from build123d import *

# Parameters (mm, degrees)
SKETCH1_R           = 5.0927
BOSS_EXTRUDE1_DEPTH = 5.2578
SKETCH2_R           = 2.3495
CUT_EXTRUDE1_DEPTH  = 9.917154671
SKETCH3_R           = 4.2037
CUT_EXTRUDE2_DEPTH  = 4.4958
CUT_EXTRUDE3_DEPTH  = 4.4958
BOSS_EXTRUDE2_START = 2.54
BOSS_EXTRUDE2_DEPTH = 2.54


with BuildPart() as part:
    # Sketch1 → Boss-Extrude1 (new body)
    with BuildSketch(Plane(origin=(0, 0, 0), x_dir=(1, 0, 0), z_dir=(0, 1, 0))):
        with Locations(Location((0, 0, 0), (0, 0, 270))):
            Circle(SKETCH1_R)
    extrude(amount=BOSS_EXTRUDE1_DEPTH)

    # Sketch2 → Cut-Extrude1 (cut, through all)
    with BuildSketch(Plane(origin=(0, 5.2578, 0), x_dir=(1, 0, 0), z_dir=(0, 1, 0))):
        with Locations(Location((0, 0, 0), (0, 0, 270))):
            Circle(SKETCH2_R)
    extrude(amount=-CUT_EXTRUDE1_DEPTH, mode=Mode.SUBTRACT)

    # Sketch3 → Cut-Extrude2 (cut)
    with BuildSketch(Plane.XZ):
        with Locations(Location((0, 0, 0), (0, 0, 270))):
            Circle(SKETCH3_R)
    extrude(amount=-CUT_EXTRUDE2_DEPTH, mode=Mode.SUBTRACT)

    # Sketch5 → Cut-Extrude3 (cut)
    with BuildSketch(Plane.XZ):
        with BuildLine():
            Line((0, 0), (4.51728007, 2.351547163))
            ThreePointArc((4.51728007, 2.351547163), (0, 5.0927), (-4.51728007, 2.351547163))
            Line((-4.51728007, 2.351547163), (0, 0))
        make_face()
    extrude(amount=-CUT_EXTRUDE3_DEPTH, mode=Mode.SUBTRACT)

    # Sketch4 → Boss-Extrude2 (add)
    with BuildSketch(Plane(origin=(0, 5.2578, 0), x_dir=(1, 0, 0), z_dir=(0, 1, 0)).offset(BOSS_EXTRUDE2_START)):
        with BuildLine():
            Line((4.332897797, 4.7285282), (1.587299193, 1.732233103))
            ThreePointArc((1.587299193, 1.732233103), (-0.306671289, 2.329399702), (-1.981548202, 1.26238543))
            Line((-1.981548202, 1.26238543), (-5.409091038, 3.445971038))
            ThreePointArc((-5.409091038, 3.445971038), (-0.837129734, 6.358631618), (4.332897797, 4.7285282))
        make_face()
    extrude(amount=-BOSS_EXTRUDE2_DEPTH)


solid = part.part
Input: part model. Units: mm. Frame: model coordinates. A direction names the side the tool comes from. Give positions to 0.01 mm unless a question says otherwise; leave off trailing zeros. Write each loop counter-clockwise with the first axis right and the second up, starting at its lowest first coordinate (ties: lowest second). Pieces come first, ordered by that corner, then holes.
Q1. Pull-direction query (X, two-part tool) for faces 6 (the face through (-0.91, 6.55, -6.35)), 7 (the face through (-0.12, 2.22, -4.2)), 8 (the face through (2.98, 6.55, -3.25)); classes: pulls with the +X half, pulls with the -X half, needs draft (parallel to the pull), parting line crosses it, or undercut.
Q2. Set-up query: faces 1 (the face through (-3.67, 6.55, -2.34)), 2 (the face through (-3.1, 2.59, -4.04)), 3 (the face through (0, 7.798, -4)), 4 (the face through (0, 0, -4.4)), 5 (the face through (-0.5, 5.258, -5.3)). Return all of +Z, -Z, +X, -X, +Y, -Y with unobstructed straight access to the full face (end or side cutting, diameter ignored); none if empty.
Q3. Section A-A, the plane z = 0. Output: boundary loops of the cut face in (x, y).
Q4. First-contact query: P1, Ø3, axis at x = 3.5, y = 4.5, coming from the -Z side; P2, Ø2, axis at y = 5.5, z = -1, coming from the -X side; P3, Ø2, axis at x = -1, y = 4, coming from the +Z side. Flat tips, straight axial feed; report the tip coordinate or a pass-through.
Q5. Section C-C, the plane x = -2.5. Output: boundary loops of the cut face in (y, z).
Q6. Section D-D, the plane y = 2.25. Output: boundary loops of the cut face in (x, z), plus the area to 3 significant figures.
Q7. Section B-B, the plane x = 0. Output: boundary loops of the cut face in (y, z).
Q8. Material intervals for probe 1 along Z at (x, y) = (0, 4.85); probe 2 along X at (y, z) = (2.85, 0), sorted ascending.
Filled in:
1. face 6: parting line crosses it
1. face 7: undercut
1. face 8: pulls with the +X half
2. face 1: +Z, -X, +Y
2. face 2: -Y
2. face 3: +Z, -Z, +X, -X, +Y
2. face 4: +Z, -Z, +X, -X, -Y
2. face 5: -Z, -Y
3. outline: (-5.09, 0) - (-4.2, 0) - (-4.2, 4.5) - (-2.35, 4.5) - (-2.35, 5.26) - (-5.09, 5.26) - close; (2.35, 4.5) - (4.2, 4.5) - (4.2, 0) - (5.09, 0) - (5.09, 5.26) - (2.35, 5.26) - close
4. P1: stops at z = -6.02
4. P2: stops at x = -5.09
4. P3: stops at z = 5.09
5. outline: (0, -4.44) - (5.26, -4.44) - (5.26, -5.91) - (7.8, -5.91) - (7.8, -1.59) - (5.26, -1.59) - (5.26, 4.44) - (4.5, 4.44) - (4.5, -3.38) - (0, -3.38) - close
6. outline: (-4.52, 2.35) arc R5.09 ccw (long way) to (4.52, 2.35) - (3.73, 1.94) arc R4.2 cw (long way) to (-3.73, 1.94) - close
6. area: 16.9 mm2
7. outline: (0, -5.09) - (5.26, -5.09) - (5.26, -6.41) - (7.8, -6.41) - (7.8, -2.35) - (4.5, -2.35) - (4.5, -4.2) - (0, -4.2) - close; (4.5, 2.35) - (5.26, 2.35) - (5.26, 5.09) - (4.5, 5.09) - close
8. probe 1: z = -5.09 to -2.35, 2.35 to 5.09
8. probe 2: x = -5.09 to -4.2, 4.2 to 5.09
